from build123d import *

# Parameters (mm, degrees)
SKETCH1_R           = 3.75
SKETCH1_R_2         = 2.25
BOSS_EXTRUDE2_DEPTH = 2.25
FILLET1_R           = 0.5


with BuildPart() as part:
    # Sketch1 → Boss-Extrude2 (new, symmetric)
    with BuildSketch(Plane.XY.offset(58)):
        with Locations((-4.039970845, 19.325746234)):
            Circle(SKETCH1_R)
        with Locations((-4.039970845, 19.325746234)):
            Circle(SKETCH1_R_2, mode=Mode.SUBTRACT)
    extrude(amount=BOSS_EXTRUDE2_DEPTH, both=True)

    # Fillet1
    fillet1_edges = [part.edges().sort_by_distance(p)[0] for p in [
        (-7.789970845, 19.325746234, 55.75),
        (-7.789970845, 19.325746234, 60.25),
        (-6.289970845, 19.325746234, 55.75),
        (-6.289970845, 19.325746234, 60.25),
    ]]
    fillet(fillet1_edges, radius=FILLET1_R)


solid = part.part
Verification items for the finished model (mm, model axes). Give positions to 0.01 mm unless a question says otherwise; leave off trailing zeros. Loops run counter-clockwise (first coordinate to the right, second up) from the corner with the lowest first, then second, coordinate; pieces in that order, holes last.
1. Material ranges on probe 1 along Y at (x, z) = (-4, 56.4); probe 2 along Y at (x, z) = (-4.5, 57.65); probe 3 along X at (y, z) = (18.25, 60.15), recorded low to high.
Derived:
probe 1: y = 15.58 to 17.08, 21.58 to 23.08
probe 2: y = 15.6 to 17.12, 21.53 to 23.05
probe 3: x = -7.42 to -6.24, -1.84 to -0.66
2. Release check for a two-part mould opening along X. For faces 1 (the cylindrical face through (-4.853, 15.665, 58.024)), 2 (the flat face through (-7, 20, 55.75)), 3 (the cylindrical face through (-4.53, 17.13, 57.98)) record: +X half, -X half, draft (parallel to the pull), parting line (faces both ways), or undercut.
Derived:
face 1: parting line
face 2: draft
face 3: undercut
3. Go/stop test with flat-tipped pins: P1, Ø2, axis at y = 22, z = 58, coming from the -X side; P2, Ø1.5, axis at x = -1.5, z = 57, coming from the +Y side. Record where each tip stops, or that it passes through.
Derived:
P1: stops at x = -7.4
P2: stops at y = 22.62
4. Cross-section at A-A on z = 59.1. Record the cut outline in (x, y), and give its area (3 significant figures).
Derived:
outline: circle Ø7.5 at (-4.04, 19.33); hole circle Ø4.5 at (-4.04, 19.33)
area: 28.3 mm2
